```python
from build123d import *

# Parameters (mm, degrees)
SKETCH_2_R          = 12.5
SKETCH_2_R_2        = 6.75
EXTRUDE_1_DEPTH     = 2
SKETCH_3_R          = 1.55
CUT_EXTRUDE_1_DEPTH = 18.790446875


with BuildPart() as part:
    # 草图2 → 凸台-拉伸1 (new body)
    with BuildSketch(Plane(origin=(0, 0, 0), x_dir=(1, 0, 0), z_dir=(0, 1, 0))):
        with Locations(Location((0, 0, 0), (0, 0, 270))):
            Circle(SKETCH_2_R)
        with Locations(Location((0, 0, 0), (0, 0, 270))):
            Circle(SKETCH_2_R_2, mode=Mode.SUBTRACT)
    extrude(amount=EXTRUDE_1_DEPTH)

    # 草图3 → 切除-拉伸1 (cut, through all)
    with BuildSketch(Plane(origin=(0, 2, 0), x_dir=(1, 0, 0), z_dir=(0, 1, 0))):
        with Locations(Location((0, 9.5, 0), (0, 0, 270))):
            Circle(SKETCH_3_R)
        with Locations(Location((8.227241336, -4.75, 0), (0, 0, 270))):
            Circle(SKETCH_3_R)
        with Locations(Location((-8.227241336, -4.75, 0), (0, 0, 270))):
            Circle(SKETCH_3_R)
    extrude(amount=-CUT_EXTRUDE_1_DEPTH, mode=Mode.SUBTRACT)


solid = part.part
```
Read the model definition and answer for the solid it produces. Units are mm, in the model's axes. Round coordinates to 2 decimals unless told otherwise and drop trailing zeros. Write each loop counter-clockwise with the first axis right and the second up, starting at its lowest first coordinate (ties: lowest second). Pieces come first, ordered by that corner, then holes. Notation, with made-up numbers: M -36.75,53 L -22.75,53 A35 ccw -22.75,89 Z; hole C -38.5,59 d10. An arc over 180 degrees is marked long. One line per item, written item: value.
Q1. Find section D-D on y = 0.6. Write down the section's boundary in (x, z), plus the area to 3 significant figures.
Data:
outline: C 0,0 d25; hole C -8.23,4.75 d3.1; hole C 0,0 d13.5; hole C 0,-9.5 d3.1; hole C 8.23,4.75 d3.1
area: 325 mm2
Q2. Find section B-B on x = 0. Write down the section's boundary in (y, z), plus the area to 3 significant figures.
Data:
outline: M 0,-12.5 L 2,-12.5 L 2,-11.05 L 0,-11.05 Z; M 0,-7.95 L 2,-7.95 L 2,-6.75 L 0,-6.75 Z; M 0,6.75 L 2,6.75 L 2,12.5 L 0,12.5 Z
area: 16.8 mm2
Q3. For a pull along Z with two mould halves and no side action, classify faces 1 (the cylindrical face through (-6.59, 0.99, -1.46)), 2 (the cylindrical face through (-8.2, 1, 3.2)), 3 (the cylindrical face through (3.755, 0.986, 11.923)), 4 (the flat face through (-5, 2, 5)) as +Z half, -Z half, draft (parallel to the pull), parting line (faces both ways), or undercut.
Data:
face 1: undercut
face 2: undercut
face 3: parting line
face 4: draft
Q4. Find section A-A on z = 0. Write down the section's boundary in (x, y), plus the area to 3 significant figures.
Data:
outline: M -12.5,0 L -6.75,0 L -6.75,2 L -12.5,2 Z; M 6.75,0 L 12.5,0 L 12.5,2 L 6.75,2 Z
area: 23.0 mm2
Q5. Find section C-C on z = 4.75. Write down the section's boundary in (x, y).
Data:
outline: M -11.56,0 L -9.78,0 L -9.78,2 L -11.56,2 Z; M -6.68,0 L -4.8,0 L -4.8,2 L -6.68,2 Z; M 4.8,0 L 6.68,0 L 6.68,2 L 4.8,2 Z; M 9.78,0 L 11.56,0 L 11.56,2 L 9.78,2 Z
Q6. Straight lines are drawn through the part: line 1 (X direction, y = 1.05, z = 0); line 2 (Z direction, x = -0.75, y = 1.7); line 3 (X direction, y = 0.5, z = 3.75). For each, find the intervals that lie inside material, in ascending order. Write a range as [from, to].
Data:
line 1: [-12.5, -6.75], [6.75, 12.5]
line 2: [-12.48, -10.86], [-8.14, -6.71], [6.71, 12.48]
line 3: [-11.92, -9.41], [-7.04, -5.61], [5.61, 7.04], [9.41, 11.92]
